Solid Edge part; units mm, degrees
sketch "Sketch1" plane through (0, 0, 0) normal (0, 0, 1) x (1, 0, 0)
  circle A0 centre (0, 0) radius 17.4
extrude "Protrusion1" add sketch "Sketch1" along normal blind 12.88
sketch "Sketch2" plane through (0, 0, 0) normal (0, 0, -1) x (1, 0, 0)
  circle A0 centre (0, 0) radius 10
extrude "Protrusion2" add sketch "Sketch2" along normal blind 115
sketch "Sketch3" plane through (0, 0, -115) normal (0, 0, -1) x (1, 0, 0)
  circle A0 centre (0, 0) radius 9.9997
extrude "Cutout1" cut sketch "Sketch3" against normal blind 46 flip side to cut
chamfer "Chamfer_1" distance 1.5 angle 45 1 edges at (-9.9997, 0, -115)
sketch "Sketch4" plane through (0, 0, 12.88) normal (0, 0, 1) x (1, 0, 0)
  line L0 (-8.8182, 15) -> (8.8182, 15)
extrude "Cutout2" cut sketch "Sketch4" against normal up to next material side at (0, 15.05, 12.88)
pattern_circular "Pattern1" count 6 over 360 about axis through (0, 0, 12.88) along (0, 0, 1) of "Cutout2"
properties part number "160787"
The listing builds one solid part. Answer for the finished solid, in the listing's coordinates (mm). A direction names the side the tool comes from. Give positions to 0.01 mm unless a question says otherwise; leave off trailing zeros. Order: outer loops, then holes, each group sorted by start corner. A loop starts at its lowest first (then second) coordinate and runs counter-clockwise, first axis right, second up. Notation, with made-up numbers: M 2.5,74 L 50.5,74 A18 ccw 50.5,99 Z; hole C -18,23.5 d8. An arc over 180 degrees is marked long. Put each result on its own line as item: value. Start each with the question number.
Item 1: The part is cut by section C-C, the plane z = -73. Determine the outline of the cut face in (x, y), and give its area (3 significant figures).
Item 2: The part is cut by section B-B, the plane z = 2. Determine the outline of the cut face in (x, y).
Item 3: Which of the six approach directions +Z, -Z, +X, -X, +Y, -Y give full straight-line access (tool end or side, diameter ignored) to faces 4 (the face through (-2.17, -9.76, -34.02)), 5 (the face through (-13.05, 7.4, 6.53))?
Item 4: Flat-ended cylindrical pins translate along their axes: P1, Ø1, axis at y = 3, z = -59.5, coming from the +X side; P2, Ø5, axis at y = 2.5, z = -89, coming from the +X side; P3, Ø5, axis at x = 5, z = -19, coming from the -Y side; P4, Ø8, axis at x = -6.5, y = 9.5, coming from the -Z side. Find the tip coordinate at first contact, or state that the pin passes through.
Item 5: For a pull along X with two mould halves and no side action, classify faces 1 (the face through (0, 15, 7)), 2 (the face through (-2.17, 9.76, -91.56)), 3 (the face through (12.93, 7.605, 6.53)) as +X half, -X half, draft (parallel to the pull), parting line (faces both ways), or undercut.
Item 6: Find the intervals of material crossed by line 1 along X through (y, z) = (-0.5, -38.5); line 2 along Z through (x, y) = (-10, 8.5); line 3 along X through (y, z) = (-5, -109), in increasing order.
Answer key:
1. outline: C 0,0 d20
1. area: 314 mm²
2. outline: M -17.32,0 L -8.66,-15 L 8.66,-15 L 17.32,0 L 8.66,15 L -8.66,15 Z
3. face 4: -Z
3. face 5: +Z, -Z, -X, +Y
4. P1: stops at x = 9.68
4. P2: stops at x = 10
4. P3: stops at y = -9.68
4. P4: stops at z = -115
5. face 1: draft
5. face 2: parting line
5. face 3: +X half
6. line 1: x = -9.99 to 9.99
6. line 2: z = 0 to 12.88
6. line 3: x = -8.66 to 8.66
